For this review, take the finished solid that the model builds, in its own axes (mm). A direction names the side the tool comes from. Coordinates: 2 decimals unless noted, no trailing zeros. Write each loop counter-clockwise with the first axis right and the second up, starting at its lowest first coordinate (ties: lowest second). Pieces come first, ordered by that corner, then holes. Notation, with made-up numbers: M 2.5,10 L 21.5,10 A22 cw 21.5,38 Z; hole C -1,18 d6. An arc over 180 degrees is marked long. Return JSON: item names as keys, results as strings.
```python
from build123d import *

# Parameters (mm, degrees)
BOSS_EXTRU_1_DEPTH      = 45
ENL_V_MAT_EXTRU_1_DEPTH = 609.201213002
ESQUISSE3_R             = 2
ENL_V_MAT_EXTRU_2_DEPTH = 91.138958208
ESQUISSE4_R             = 3
ENL_V_MAT_EXTRU_3_DEPTH = 46.15


with BuildPart() as part:
    # Esquisse1 → Boss.-Extru.1 (new body)
    with BuildSketch(Plane.XY):
        Polygon((-38, -554.760879723), (-38, -596.760879723), (0, -596.760879723), (0, -605.060879723), (-59.74898984, -605.060879723), (-59.74898984, -600.910879723), (-42.249820419, -596.760879723), (-42.249820419, -554.760879723), align=None)
    extrude(amount=-BOSS_EXTRU_1_DEPTH)

    # Esquisse2 → Enlèv. mat.-Extru.1 (cut, through all)
    with BuildSketch(Plane.ZY.offset(42.249820419)):
        with BuildLine():
            ThreePointArc((-12.006985294, -576.988423193), (-4.2, -575.760879723), (-12.006985294, -574.533336253))
            ThreePointArc((-12.006985294, -574.533336253), (-38.45, -575.760879723), (-12.006985294, -576.988423193))
        make_face()
    extrude(amount=-ENL_V_MAT_EXTRU_1_DEPTH, mode=Mode.SUBTRACT)

    # Esquisse3 → Enlèv. mat.-Extru.2 (cut, through all)
    with BuildSketch(Plane.XZ.offset(605.060879723)):
        with Locations(Location((-50.683510071, -35, 0), (0, 0, 270))):
            Circle(ESQUISSE3_R)
        with Locations(Location((-50.683510071, -10, 0), (0, 0, 270))):
            Circle(ESQUISSE3_R)
    extrude(amount=-ENL_V_MAT_EXTRU_2_DEPTH, mode=Mode.SUBTRACT)

    # Esquisse4 → Enlèv. mat.-Extru.3 (cut)
    with BuildSketch(Plane(origin=(0, -554.760879723, 0), x_dir=(1, 0, 0), z_dir=(0, 1, 0))):
        with Locations(Location((-50.683510071, 10, 0), (0, 0, 270))):
            Circle(ESQUISSE4_R)
        with Locations(Location((-50.683510071, 35, 0), (0, 0, 270))):
            Circle(ESQUISSE4_R)
    extrude(amount=-ENL_V_MAT_EXTRU_3_DEPTH, mode=Mode.SUBTRACT)


solid = part.part
```
1. We need section C-C (z = -34). State the section outline as (x, y) points.
Checks:
{"outline": "M -59.75,-605.06 L -52.42,-605.06 L -52.42,-600.91 L -53.51,-600.91 L -53.51,-599.43 L -59.75,-600.91 Z; M -48.95,-605.06 L 0,-605.06 L 0,-596.76 L -38,-596.76 L -38,-585.67 L -42.25,-585.67 L -42.25,-596.76 L -47.86,-598.09 L -47.86,-600.91 L -48.95,-600.91 Z; M -42.25,-565.86 L -38,-565.86 L -38,-554.76 L -42.25,-554.76 Z"}
2. For faces 1 (the face through (-38, -580, -12)), 2 (the face through (-42.25, -581, -12)), 3 (the face through (-53, -600.911, -34)), 4 (the face through (-32, -598, -45)), list the 3-axis set-ups (+Z, -Z, +X, -X, +Y, -Y) from which the entire face can be reached by the end or side of a thin tool; tool diameter is ignored.
Checks:
{"face 1": "+Z, -Z, +X, +Y", "face 2": "+Z, -Z, -X, +Y", "face 3": "+Y", "face 4": "-Z, +X, -X, +Y, -Y"}
3. Clearance check with flat-ended pins moving along their axes: pin 1 Ø5 at (y, z) = (-568, -16.5) entering from +X; pin 2 Ø11.5 at (x, z) = (-23.5, -20) entering from +Y; pin 3 Ø3 at (x, z) = (-52, -36) entering from +Y. State where each tip first meets the part, or that it passes through.
Checks:
{"pin 1": "x = -38", "pin 2": "y = -596.76", "pin 3": "y = -599.18"}
4. Draft analysis for pull direction Y (two halves, no side actions). For faces 5 (the face through (-29, -605.061, -22)), 6 (the face through (-40.15, -575.2, -38.44)), 7 (the face through (-52.46, -603.01, -10.92)), 8 (the face through (-40.155, -575.919, -4.203)), state which applies: +Y half, -Y half, draft (parallel to the pull), parting line (faces both ways), or undercut.
Checks:
{"face 5": "-Y half", "face 6": "undercut", "face 7": "draft", "face 8": "undercut"}
5. Wall thickness on L1, parallel to X at y = -603.8, z = -10; L2, parallel to Y at x = -8.5, z = -6.5; L3, parallel to X at y = -581, z = -42: over which ranges is each line inside the solid? List them lowest first. Write a range as from..to.
Checks:
{"L1": "-59.75..-52.68, -48.68..0", "L2": "-605.06..-596.76", "L3": "-42.25..-38"}
6. We need section A-A (z = -25.2). State the section outline as (x, y) points.
Checks:
{"outline": "M -59.75,-605.06 L 0,-605.06 L 0,-596.76 L -38,-596.76 L -38,-589.01 L -42.25,-589.01 L -42.25,-596.76 L -59.75,-600.91 Z; M -42.25,-562.51 L -38,-562.51 L -38,-554.76 L -42.25,-554.76 Z"}
7. We need section B-B (y = -586). State the section outline as (x, z) points.
Checks:
{"outline": "M -42.25,-45 L -38,-45 L -38,-33.61 L -42.25,-33.61 Z; M -42.25,-16.79 L -38,-16.79 L -38,0 L -42.25,0 Z"}
8. We need section D-D (x = -29.5). State the section outline as (y, z) points, plus the area to 4 significant figures.
Checks:
{"outline": "M -605.06,-45 L -596.76,-45 L -596.76,0 L -605.06,0 Z", "area": "373.5 mm2"}
